Work out the finished part from the listing and answer in its coordinate system (mm). A direction names the side the tool comes from. Round coordinates to 2 decimals unless told otherwise and drop trailing zeros. Loops run counter-clockwise (first coordinate to the right, second up) from the corner with the lowest first, then second, coordinate; pieces in that order, holes last. Notation, with made-up numbers: (0.25, 17) -> (17.25, 17) arc R26 ccw to (17.25, 52) -> close; hole circle Ø6 at (83, -27.5). An arc over 180 degrees is marked (long way). Use CSV: the item, a comma, the result in double quotes. Start each with the question number.
from build123d import *

# Parameters (mm, degrees)
F0_W         = 152.4
F0_H         = 152.4
F0_W_2       = 101.6
F0_H_2       = 101.6
F1_DEPTH     = 25.4
F2_W         = 152.4
F2_H         = 152.4
F2_W_2       = 101.6
F2_H_2       = 101.6
F1_FACE1_W   = 152.4
F1_FACE1_H   = 152.4
F1_FACE1_W_2 = 101.6
F1_FACE1_H_2 = 101.6
F3_DEPTH     = 25.4
F4_DEPTH     = 25.4
F6_DEPTH     = 65.9318938851


with BuildPart() as f1:
    # F0 (on Front) → F1 (new body)
    with BuildSketch(Plane.XZ):
        with Locations((-37.793815136, -33.3924548149)):
            Rectangle(F0_W, F0_H)
        with Locations((-37.793815136, -33.3924548149)):
            Rectangle(F0_W_2, F0_H_2, mode=Mode.SUBTRACT)
    extrude(amount=F1_DEPTH)

    # F2 (on face) + F1_face1 (on face) → F3 (join)
    with BuildSketch(Plane.XZ.offset(25.4)):
        with Locations((-37.793815136, -33.3924548149)):
            Rectangle(F2_W, F2_H)
        with Locations((-37.793815136, -33.3924548149)):
            Rectangle(F2_W_2, F2_H_2, mode=Mode.SUBTRACT)
    with BuildSketch(Plane(origin=(-37.793815136, 0, -33.3924548149), x_dir=(1, 0, 0), z_dir=(0, 1, 0))):
        Rectangle(F1_FACE1_W, F1_FACE1_H)
        Rectangle(F1_FACE1_W_2, F1_FACE1_H_2, mode=Mode.SUBTRACT)
    extrude(amount=F3_DEPTH, dir=(0, -1, 0))

    # F4 (add): a face of the model
    f4_faces = [f1.faces().sort_by_distance(p)[0] for p in [
        (-37.793815136, -25.4, -109.5924548149),
    ]]
    extrude(f4_faces, amount=F4_DEPTH)

    # F5 (on face) → F6 (join)
    with BuildSketch(Plane(origin=(0, 0, -134.9924548149), x_dir=(1, 0, 0), z_dir=(0, 0, -1))):
        with BuildLine():
            ThreePointArc((-38.6654032298, 0), (-38.7976029218, 0.6748576376), (-38.9661378476, 1.3415701457))
            ThreePointArc((-38.9661378476, 1.3415701457), (-40.2086037303, 0.632175677), (-41.4920817767, 0))
            Line((-41.4920817767, 0), (-38.6654032298, 0))
        make_face()
        with BuildLine():
            ThreePointArc((-38.9661378476, 1.3415701457), (-51.1900559068, 10.5968891325), (-63.4139739659, 1.3415701457))
            ThreePointArc((-63.4139739659, 1.3415701457), (-62.1715080832, 0.632175677), (-60.8880300369, 0))
            Line((-60.8880300369, 0), (-41.4920817767, 0))
            ThreePointArc((-41.4920817767, 0), (-40.2086037303, 0.632175677), (-38.9661378476, 1.3415701457))
        make_face()
        with BuildLine():
            ThreePointArc((-60.8880300369, 0), (-62.1715080832, 0.632175677), (-63.4139739659, 1.3415701457))
            ThreePointArc((-63.4139739659, 1.3415701457), (-63.5825088917, 0.6748576376), (-63.7147085837, 0))
            Line((-63.7147085837, 0), (-60.8880300369, 0))
        make_face()
        with BuildLine():
            ThreePointArc((-41.4920817767, 0), (-51.1900559068, -2.1031108675), (-60.8880300369, 0))
            Line((-60.8880300369, 0), (-63.7147085837, 0))
            ThreePointArc((-63.7147085837, 0), (-52.2452599161, -14.7591981183), (-38.4900559068, -2.1031108675))
            ThreePointArc((-38.4900559068, -2.1031108675), (-38.533968656, -1.0479068583), (-38.6654032298, 0))
            Line((-38.6654032298, 0), (-41.4920817767, 0))
        make_face()
        with BuildLine():
            Line((-41.4920817767, 0), (-60.8880300369, 0))
            ThreePointArc((-60.8880300369, 0), (-51.1900559068, -2.1031108675), (-41.4920817767, 0))
        make_face()
        with BuildLine():
            ThreePointArc((-38.9661378476, 1.3415701457), (-30.7660990603, 9.8646449948), (-27.7785993191, 21.3083457202))
            ThreePointArc((-27.7785993191, 21.3083457202), (-62.6337566322, 41.7323025666), (-63.4139739659, 1.3415701457))
            ThreePointArc((-63.4139739659, 1.3415701457), (-51.1900559068, 10.5968891325), (-38.9661378476, 1.3415701457))
        make_face()
    extrude(amount=-F6_DEPTH)


solid = f1.part
Q1. Which of the six approach directions +Z, -Z, +X, -X, +Y, -Y give full straight-line access (tool end or side, diameter ignored) to faces 4 (the flat face through (-39, -25, 17.408)), 5 (the flat face through (-38.9, -50.8, -84.4))?
Q2. Section B-B, the plane z = -15 is taken. Write down the section's boundary in (x, y).
Q3. For a pull along Z with two mould halves and no side action, classify faces 1 (the flat face through (38.406, -25, -45)), 2 (the flat face through (-39, -25, 42.808)), 3 (the flat face through (13.006, -25, -34)) as pulls with the +Z half, pulls with the -Z half, needs draft (parallel to the pull), parting line crosses it, or undercut.
Q4. Straight lines are drawn through the part: line 1 (X direction, y = -32, z = -24); line 2 (Z direction, x = 10, y = -37); line 3 (Z direction, x = -67.5, y = -27.5). For each, find the intervals that lie inside material, in ascending order. Write a range as from..to.
Q5. Section C-C, the plane y = -41 is taken. Write down the section's boundary in (x, z).
Q6. Section D-D, the plane z = -117 is taken. Write down the section's boundary in (x, y), and give its area (3 significant figures).
Q7. Section A-A, the plane x = -83 is taken. Write down the section's boundary in (y, z), and give its area (3 significant figures).
Report:
1,face 4,"+Y, -Y"
1,face 5,"+Z, -Z, +X, -X, -Y"
2,outline,"(-113.99, -50.8) -> (-88.59, -50.8) -> (-88.59, 0) -> (-113.99, 0) -> close; (13.01, -50.8) -> (38.41, -50.8) -> (38.41, 0) -> (13.01, 0) -> close"
3,face 1,"needs draft"
3,face 2,"pulls with the +Z half"
3,face 3,"undercut"
4,line 1,"x = -113.99..-88.59, 13.01..38.41"
4,line 2,"z = -134.99..-84.19, 17.41..42.81"
4,line 3,"z = -134.99..-69.06, 17.41..42.81"
5,outline,"(-113.99, -134.99) -> (38.41, -134.99) -> (38.41, 42.81) -> (-113.99, 42.81) -> close; hole (-88.59, -84.19) -> (-63.85, -84.19) -> (-63.85, -69.06) -> (-38.53, -69.06) -> (-38.53, -84.19) -> (13.01, -84.19) -> (13.01, 17.41) -> (-88.59, 17.41) -> close"
6,outline,"(-113.99, -50.8) -> (38.41, -50.8) -> (38.41, 0) -> (-38.67, 0) arc R12.7 ccw (long way) to (-63.71, 0) -> (-113.99, 0) -> close"
6,area,"8,050 mm²"
7,outline,"(-50.8, -134.99) -> (0, -134.99) -> (0, -84.19) -> (-50.8, -84.19) -> close; (-50.8, 17.41) -> (0, 17.41) -> (0, 42.81) -> (-50.8, 42.81) -> close"
7,area,"3,870 mm²"
